CAD build for the part. Positions are in the model's coordinates, mm. Face numbers are marked on the shaded views. A direction names the side the tool comes from. Coordinates: 2 decimals unless noted, no trailing zeros. Loops run counter-clockwise (first coordinate to the right, second up) from the corner with the lowest first, then second, coordinate; pieces in that order, holes last. Notation, with made-up numbers: (77.5, 23.25) - (84.5, 23.25) arc R5 cw to (84.5, 30.25) - close; hole circle Ø6 at (11, -32). An arc over 180 degrees is marked (long way). Put each result on its own line as item: value.
```python
from build123d import *

# Parameters (mm, degrees)
EXTRUDE_1_DEPTH     = 4.5
EXTRUDE_5_DEPTH     = 19.5
EXTRUDE_6_DEPTH     = 20
EXTRUDE_7_DEPTH     = 5
SKETCH_6_R          = 2.6
CUT_EXTRUDE_1_DEPTH = 36.209916548
SKETCH_13_R         = 2.6
CUT_EXTRUDE_2_DEPTH = 41.493681277
FILLET_1_R          = 2.5
FILLET_2_R          = 10


with BuildPart() as part:
    # Эскиз1 → Бобышка-Вытянуть1 (new body)
    with BuildSketch(Plane.XY):
        Polygon((10, 10), (-10, 10), (-10, -10), (10, -15.358983849), align=None)
    extrude(amount=EXTRUDE_1_DEPTH)

    # Эскиз10 → Бобышка-Вытянуть5 (add)
    with BuildSketch(Plane(origin=(0, 0, 0), x_dir=(-1, 0, 0), z_dir=(0, 0, -1))):
        Polygon((15, 10), (15, -13.660254038), (-10, -20.358983849), (-10, -15.358983849), (10, -10), (10, 10), align=None)
    extrude(amount=-EXTRUDE_5_DEPTH)

    # Эскиз11 → Бобышка-Вытянуть6 (add)
    with BuildSketch(Plane(origin=(0, 0, 0), x_dir=(-1, 0, 0), z_dir=(0, 0, -1))):
        Polygon((15, 10), (10, 10), (10, -15), (15, -13.660254038), align=None)
    extrude(amount=EXTRUDE_6_DEPTH)

    # Эскиз12 → Бобышка-Вытянуть7 (add)
    with BuildSketch(Plane.XY.offset(19.5)):
        Polygon((-15, -13.660254038), (10, -20.358983849), (10, 10), (-15, 10), align=None)
    extrude(amount=EXTRUDE_7_DEPTH)

    # Эскиз6 → Вырез-Вытянуть1 (cut, through all)
    with BuildSketch(Plane(origin=(0, 0, 0), x_dir=(-1, 0, 0), z_dir=(0, 0, -1))):
        Circle(SKETCH_6_R)
    extrude(amount=-CUT_EXTRUDE_1_DEPTH, mode=Mode.SUBTRACT)

    # Эскиз13 → Вырез-Вытянуть2 (cut, through all)
    with BuildSketch(Plane.ZY.offset(15)):
        with Locations(Location((-10, -1.830127019, 0), (0, 0, 270))):
            Circle(SKETCH_13_R)
    extrude(amount=-CUT_EXTRUDE_2_DEPTH, mode=Mode.SUBTRACT)

    # Скругление1
    fillet_1_edges = [part.edges().sort_by_distance(p)[0] for p in [
        (10, -20.358983849, 12.25),
        (-12.5, 10, -20),
        (-12.5, -14.330127019, -20),
    ]]
    fillet(fillet_1_edges, radius=FILLET_1_R)

    # Скругление2
    fillet_2_edges = [part.edges().sort_by_distance(p)[0] for p in [
        (10, 10, 22),
        (10, 10, 2.25),
    ]]
    fillet(fillet_2_edges, radius=FILLET_2_R)


with BuildPart() as body_2:
    # Зеркальное отражение1: mirrored copy
    add(part.part.mirror(Plane.ZX))


solid = body_2.part
```
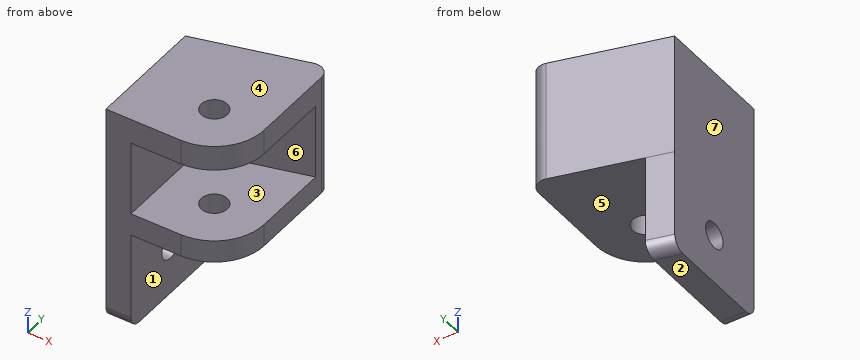
Q1. Wall check: L1, parallel to Z at x = 8.5, y = 0.75; L2, parallel to X at y = 0, z = 1.8; L3, parallel to X at y = -0.75, z = 11.5. Give the ranges that are in metal, low to high. Write a range as from..to.
Determined:
L1: 0..4.5, 19.5..24.5
L2: -15..-2.6, 2.6..10
L3: -15..-10
Q2. Pin check, flat tips, straight feed: pin 1 Ø6 at (x, y) = (3.5, -1) entering from -Z; pin 2 Ø1.5 at (y, z) = (-3.5, 7) entering from +X; pin 3 Ø12 at (y, z) = (0, 14) entering from +X; pin 4 Ø5 at (x, z) = (-0.5, 18.5) entering from +Y. Stop position of each tip, or through.
Determined:
pin 1: z = 0
pin 2: x = -10
pin 3: x = 10
pin 4: y = 18.22
Q3. Slice it at B-B, the plane x = -1.5. Give the cut face in (y, z).
Determined:
outline: (-10, 0) - (-2.12, 0) - (-2.12, 4.5) - (-10, 4.5) - close; (-10, 19.5) - (-2.12, 19.5) - (-2.12, 24.5) - (-10, 24.5) - close; (2.12, 0) - (17.28, 0) - (17.28, 24.5) - (2.12, 24.5) - (2.12, 19.5) - (12.28, 19.5) - (12.28, 4.5) - (2.12, 4.5) - close
Q4. Tool access for the marked faces 5, 6 and 7: list every direction of +Z, -Z, +X, -X, +Y, -Y with a clear straight run to the whole face (end or side of a thin tool).
Determined:
face 5: -Z, +X, +Y, -Y
face 6: +X, -Y
face 7: +Z, -Z, -X, +Y, -Y
Q5. Slice it at D-D, the plane y = 1.5. Give the cut face in (x, z), then the cut area to 3 significant figures.
Determined:
outline: (-15, -20) - (-10, -20) - (-10, -12.58) - (-15, -12.58) - close; (-15, -7.42) - (-10, -7.42) - (-10, 0) - (-2.12, 0) - (-2.12, 4.5) - (-10, 4.5) - (-10, 19.5) - (-2.12, 19.5) - (-2.12, 24.5) - (-15, 24.5) - close; (2.12, 0) - (10, 0) - (10, 4.5) - (2.12, 4.5) - close; (2.12, 19.5) - (10, 19.5) - (10, 24.5) - (2.12, 24.5) - close
area: 346 mm2
Q6. Slice it at A-A, the plane z = -10. Give the cut face in (x, y), then the cut area to 3 significant figures.
Determined:
outline: (-15, -10) - (-10, -10) - (-10, -0.77) - (-15, -0.77) - close; (-15, 4.43) - (-10, 4.43) - (-10, 15) - (-15, 13.66) - close
area: 95.7 mm2
Q7. Mould opens along Z. For the marked faces 1, 2, 3 and 4 say: +Z half, -Z half, draft (parallel to the pull), parting line (faces both ways), or undercut.
Determined:
face 1: draft
face 2: -Z half
face 3: undercut
face 4: +Z half
Q8. Slice it at C-C, the plane z = 8.5. Give the cut face in (x, y).
Determined:
outline: (-15, -10) - (-10, -10) - (-10, 10) - (10, 15.36) - (10, 17.1) arc R2.5 ccw to (6.85, 19.52) - (-15, 13.66) - close
